Design review of the part shown in the three views and the two pictorial views. Dimensions are in mm from the part's minimum x, y and z. Round coordinates to 2 decimals unless told otherwise and drop trailing zeros. Order: outer loops, then holes, each group sorted by start corner. A loop starts at its lowest first (then second) coordinate and runs counter-clockwise, first axis right, second up. Notation, with made-up numbers: M -14.75,87.25 L 14.25,87.25 A25 ccw 14.25,125.25 Z; hole C -38.5,26 d7. An arc over 180 degrees is marked long. Write item = value, one per line. Start each with the question number.
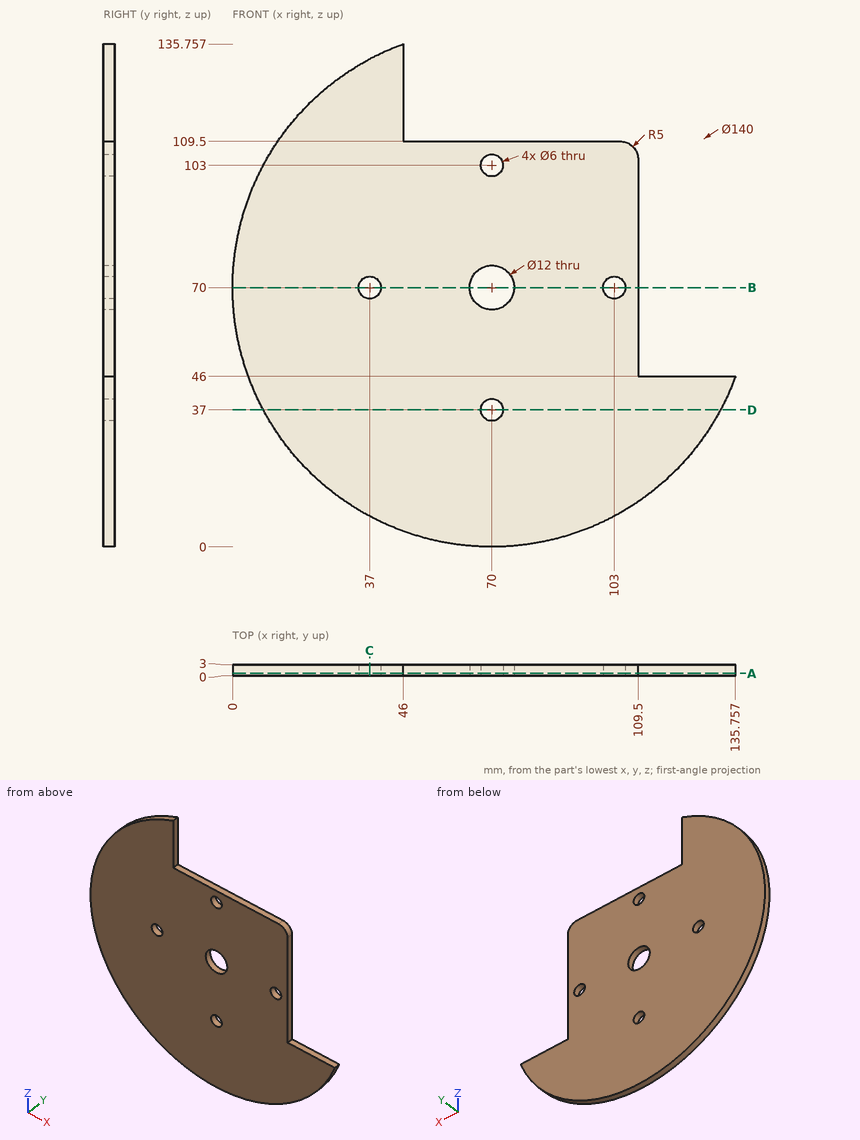
(1) We need section D-D, the plane z = 37. Write out the cut boundary in (x, y).
(2) For line 1 along X through (y, z) = (2.2, 70); line 2 along X through (y, z) = (0.65, 103), list the stretches that pass through material, from the lowest coordinate up.
(3) Insertion check: pin 1 (1 mm diameter, centred on x = 70.5, y = 2, fed in from -Z); pin 2 (1.5 mm diameter, centred on y = 1, z = 34.5, fed in from +X); pin 3 (5.5 mm diameter, centred on x = 37, z = 70, fed in from +Y); pin 4 (0.9 mm diameter, centred on x = 81, y = 2, fed in from +Z). Each pin has a flat end and moves straight along its axis. Give the tip position at first contact, or say it passes through.
(4) We need section B-B, the plane z = 70. Write out the cut boundary in (x, y).
(5) We need section C-C, the plane x = 37. Write out the cut boundary in (y, z), then the cut area to 3 significant figures.
(6) We need section A-A, the plane y = 0.7. Write out the cut boundary in (x, z).
Values:
q1.outline = M 8.27,0 L 67,0 L 67,3 L 8.27,3 Z; M 73,0 L 131.73,0 L 131.73,3 L 73,3 Z
q2.line_1 = 0 to 34, 40 to 64, 76 to 100, 106 to 109.5
q2.line_2 = 8.27 to 67, 73 to 109.5
q3.pin_1 = 0
q3.pin_2 = 130.77
q3.pin_3 = through
q3.pin_4 = 109.5
q4.outline = M 0,0 L 34,0 L 34,3 L 0,3 Z; M 40,0 L 64,0 L 64,3 L 40,3 Z; M 76,0 L 100,0 L 100,3 L 76,3 Z; M 106,0 L 109.5,0 L 109.5,3 L 106,3 Z
q5.outline = M 0,8.27 L 3,8.27 L 3,67 L 0,67 Z; M 0,73 L 3,73 L 3,131.73 L 0,131.73 Z
q5.area = 352 mm²
q6.outline = M 46,109.5 L 46,135.76 A70 ccw long 135.76,46 L 109.5,46 L 109.5,104.5 A5 ccw 104.5,109.5 Z; hole C 37,70 d6; hole C 70,70 d12; hole C 70,37 d6; hole C 70,103 d6; hole C 103,70 d6
